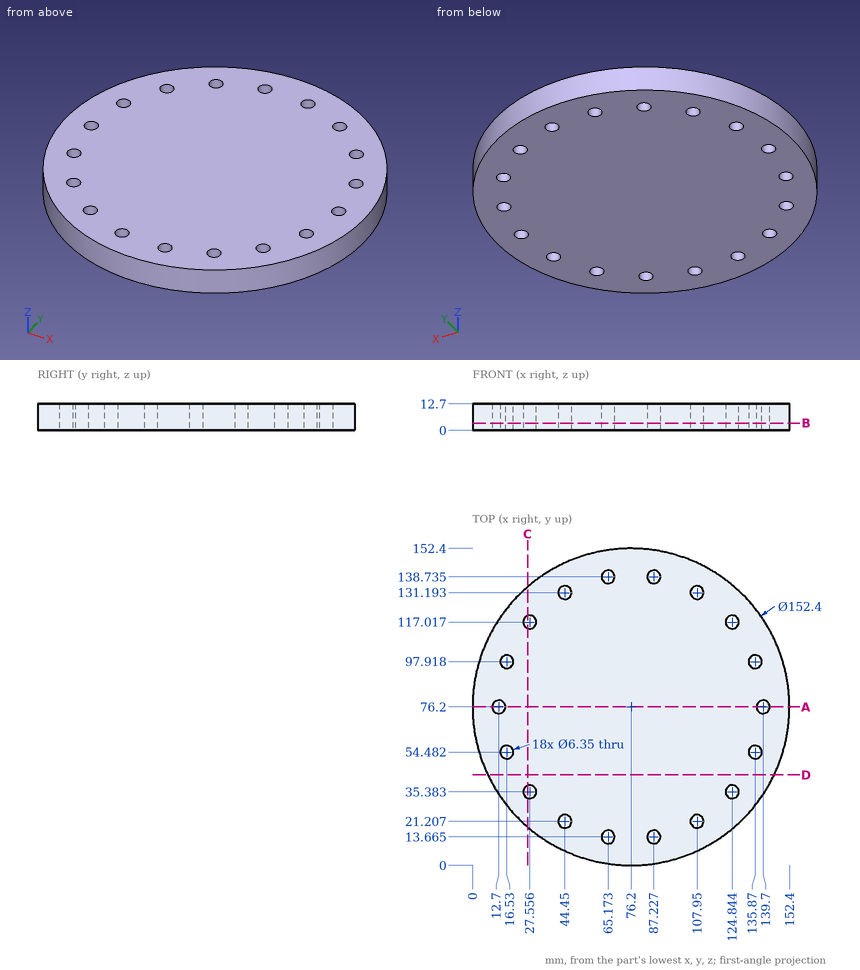
Check sheet for the drawn part. Datum: minimum x, y, z corner. Units: mm. Round coordinates to 2 decimals unless told otherwise and drop trailing zeros. Loops run counter-clockwise (first coordinate to the right, second up) from the corner with the lowest first, then second, coordinate; pieces in that order, holes last. Notation, with made-up numbers: (62.5, 53.5) - (116.5, 53.5) arc R32 cw to (116.5, 81.5) - close; hole circle Ø1 at (9.25, 2.25). An arc over 180 degrees is marked (long way). Use one line per item in the form item = value.
1. Section check B-B on z = 3.5. Give the number of separate pieces and of enclosed holes in the cut face, and give its area (3 significant figures).
A:
separate_pieces = 1
enclosed_holes = 18
area = 17,700 mm²
2. Section check C-C on x = 26.5. Record the cut outline in (y, z), and give its area (4 significant figures).
A:
outline = (18.44, 0) - (32.39, 0) - (32.39, 12.7) - (18.44, 12.7) - close; (38.38, 0) - (114.02, 0) - (114.02, 12.7) - (38.38, 12.7) - close; (120.01, 0) - (133.96, 0) - (133.96, 12.7) - (120.01, 12.7) - close
area = 1,315 mm²
3. Section check D-D on y = 43.5. Record the cut outline in (x, z), and give its area (3 significant figures).
A:
outline = (7.37, 0) - (145.03, 0) - (145.03, 12.7) - (7.37, 12.7) - close
area = 1,750 mm²
4. Gauge pin test, flat ends, axial feed: pin 1 Ø5 at (x, y) = (16.53, 97.92) entering from -Z; pin 2 Ø1.5 at (y, z) = (120.5, 6.5) entering from -X; pin 3 Ø2 at (y, z) = (59.5, 3.5) entering from -X (1 decimal); pin 4 Ø4 at (x, z) = (88.5, 4) entering from -Y. Record the tip position at first contact, or that the pin passes through.
A:
pin_1 = through
pin_2 = 13.67
pin_3 = 1.6
pin_4 = 0.7
5. Scan lines: probe 1 along X at (y, z) = (134, 12) (1 decimal); probe 2 along X at (y, z) = (136, 1) (1 decimal); probe 3 along Y at (x, z) = (85, 4.75). Record each from-to range of solid material in increasing order.
A:
probe_1 = 26.5 to 43, 45.9 to 106.5, 109.4 to 125.9
probe_2 = 29 to 63.6, 66.8 to 85.6, 88.8 to 123.4
probe_3 = 0.51 to 11.4, 15.93 to 136.47, 141 to 151.89
6. Section check A-A on y = 76.2. Record the cut outline in (x, z) (1 decimal).
A:
outline = (0, 0) - (9.5, 0) - (9.5, 12.7) - (0, 12.7) - close; (15.9, 0) - (136.5, 0) - (136.5, 12.7) - (15.9, 12.7) - close; (142.9, 0) - (152.4, 0) - (152.4, 12.7) - (142.9, 12.7) - close
